```python
from build123d import *

# Parameters (mm, degrees)
SKETCH_W              = 115
SKETCH_H              = 25
PAD_DEPTH             = 3
PAD001_DEPTH          = 3
SKETCH002_W           = 115
SKETCH002_H           = 25
SKETCH002_W_2         = 96
SKETCH002_H_2         = 3
PAD002_DEPTH          = 3
SKETCH003_R           = 1.55
POCKET_DEPTH          = 245.060315
POLARPATTERN_COUNT    = 2
POLARPATTERN001_COUNT = 2
POLARPATTERN002_COUNT = 2
FILLET_R              = 2
SKETCH004_R           = 12.75
POCKET001_DEPTH       = 3
POCKET002_DEPTH       = 3
FILLET001_R           = 0.4
FILLET002_R           = 2


with BuildPart() as part:
    # Sketch → Pad (new body)
    with BuildSketch(Plane.XY):
        Rectangle(SKETCH_W, SKETCH_H)
    extrude(amount=PAD_DEPTH)

    # Sketch001 (on Face6 of Pad) → Pad001 (join)
    with BuildSketch(Plane.XY.offset(3)):
        Polygon((-57.5, 12.5), (57.5, 12.5), (57.5, 4), (50, 4), (50, 5), (-50, 5), (-50, 4), (-57.5, 4), align=None)
        Polygon((-57.5, -12.5), (57.5, -12.5), (57.5, -4), (50, -4), (50, -5), (-50, -5), (-50, -4), (-57.5, -4), align=None)
    extrude(amount=PAD001_DEPTH)

    # Sketch002 (on Face12 of Pad001) → Pad002 (join)
    with BuildSketch(Plane.XY.offset(6)):
        Rectangle(SKETCH002_W, SKETCH002_H)
        Rectangle(SKETCH002_W_2, SKETCH002_H_2, mode=Mode.SUBTRACT)
    extrude(amount=PAD002_DEPTH)

    # Sketch003 (on Face26 of Pad002) → Pocket (cut, through all)
    with BuildSketch(Plane.XY.offset(9)):
        with Locations((-52.5, 7.5)):
            Circle(SKETCH003_R)
    pocket = extrude(amount=-POCKET_DEPTH, mode=Mode.SUBTRACT)

    # PolarPattern: Pocket ×2 about axis
    polarpattern_axis = Axis((0, 0, 0), (0, 1, 0))
    for i in range(1, POLARPATTERN_COUNT):
        add(pocket.rotate(polarpattern_axis, i * 360 / POLARPATTERN_COUNT), mode=Mode.SUBTRACT)

    # PolarPattern001: Pocket ×2 about axis
    polarpattern001_axis = Axis((0, 0, 0), (1, 0, 0))
    for i in range(1, POLARPATTERN001_COUNT):
        add(pocket.rotate(polarpattern001_axis, i * 360 / POLARPATTERN001_COUNT), mode=Mode.SUBTRACT)

    # PolarPattern002: Pocket ×2 about axis
    polarpattern002_axis = Axis((0, 0, 9), (0, 0, 1))
    for i in range(1, POLARPATTERN002_COUNT):
        add(pocket.rotate(polarpattern002_axis, i * 360 / POLARPATTERN002_COUNT), mode=Mode.SUBTRACT)

    # Fillet
    fillet_edges = [part.edges().sort_by_distance(p)[0] for p in [
        (57.5, 12.5, 7.5),
        (57.5, 12.5, 4.5),
        (57.5, 12.5, 1.5),
        (57.5, -12.5, 7.5),
        (-57.5, 12.5, 7.5),
        (-57.5, -12.5, 7.5),
    ]]
    fillet(fillet_edges, radius=FILLET_R)

    # Sketch004 (on Face2 of Fillet) → Pocket001 (cut)
    with BuildSketch(Plane(origin=(0, 0, 0), x_dir=(1, 0, 0), z_dir=(0, 0, -1))):
        with Locations((0, -4.31247)):
            Circle(SKETCH004_R)
    extrude(amount=-POCKET001_DEPTH, mode=Mode.SUBTRACT)

    # Sketch005 (on Face2 of Pocket001) → Pocket002 (cut)
    with BuildSketch(Plane(origin=(0, 0, 0), x_dir=(1, 0, 0), z_dir=(0, 0, -1))):
        Polygon((0.086598, 10.584693), (-50.025204, 10.584693), (-50.025204, 6.371434), (-55.624748, 3.161258), (-55.624748, -3.408425), (-50.493088, -3.376352), (-45.134857, 4.115264), (-43.691578, 5.783052), (0.086598, 5.783052), align=None)
    extrude(amount=-POCKET002_DEPTH, mode=Mode.SUBTRACT)

    # Fillet001
    fillet001_edges = [part.edges().sort_by_distance(p)[0] for p in [
        (-7.787357, -5.783052, 1.5),
    ]]
    fillet(fillet001_edges, radius=FILLET001_R)

    # Fillet002
    fillet002_edges = [part.edges().sort_by_distance(p)[0] for p in [
        (0.086598, -8.437236, 1.5),
    ]]
    fillet(fillet002_edges, radius=FILLET002_R)


solid = part.part
```
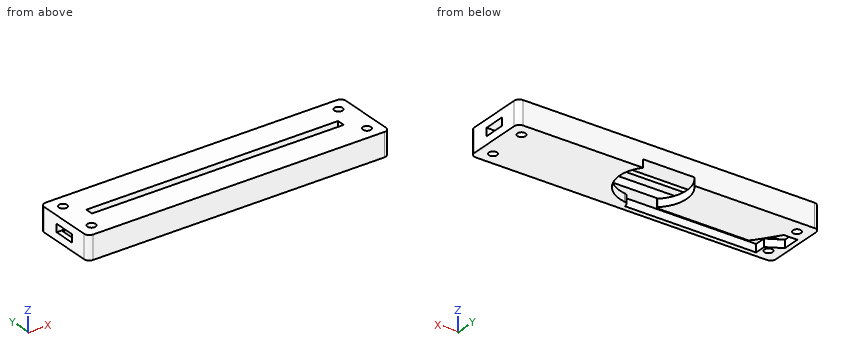
The model under review builds one solid part; all positions refer to its coordinate system, in mm. Give positions to 0.01 mm unless a question says otherwise; leave off trailing zeros. Write each loop counter-clockwise with the first axis right and the second up, starting at its lowest first coordinate (ties: lowest second). Pieces come first, ordered by that corner, then holes. Notation, with made-up numbers: M 19.5,6.25 L 44.5,6.25 A32 ccw 44.5,36.25 Z; hole C 55,24 d7. An arc over 180 degrees is marked long. Write item = value, one per line. Start each with the question number.
Q1. For line 1 (Y direction, x = 52.5, z = 7.25); line 2 (Y direction, x = 52.5, z = 5.25); line 3 (X direction, y = -7.5, z = 5.25), list the stretches that pass through material, from the lowest coordinate up.
Q2. We need section B-B (z = 7.25). State the section outline as (x, y) points, plus the area to 3 significant figures.
Q3. We need section C-C (x = -52.5). State the section outline as (y, z) points, plus the area to 3 significant figures.
Q4. We need section D-D (y = 7.5). State the section outline as (x, z) points.
Q5. We need section A-A (x = 52.5). State the section outline as (y, z) points, plus the area to 3 significant figures.
Q6. Clearance check with a flat-ended pin moving along its axis: pin 1 (8.5 mm diameter, centred on x = 0, y = 9, fed in from -Z). State where the tip first meets the part, or that it passes through.
Result set:
q1.line_1 = -12.5 to -9.05, -5.95 to 5.95, 9.05 to 12.5
q1.line_2 = -12.5 to -9.05, -5.95 to -4, 4 to 5.95, 9.05 to 12.5
q1.line_3 = -57.5 to -54.05, -50.95 to 50.95, 54.05 to 57.5
q2.outline = M -57.5,-10.5 A2 ccw -55.5,-12.5 L 55.5,-12.5 A2 ccw 57.5,-10.5 L 57.5,10.5 A2 ccw 55.5,12.5 L -55.5,12.5 A2 ccw -57.5,10.5 Z; hole C -52.5,-7.5 d3.1; hole C -52.5,7.5 d3.1; hole M -48,-1.5 L 48,-1.5 L 48,1.5 L -48,1.5 Z; hole C 52.5,-7.5 d3.1; hole C 52.5,7.5 d3.1
q2.area = 2,550 mm2
q3.outline = M -12.5,0 L -9.05,0 L -9.05,9 L -12.5,9 Z; M -5.95,0 L -4.95,0 L -4.95,3 L -4,3 L -4,6 L 4,6 L 4,3 L 3.39,3 L 3.39,0 L 5.95,0 L 5.95,9 L -5.95,9 Z; M 9.05,0 L 12.5,0 L 12.5,9 L 9.05,9 Z
q3.area = 120 mm2
q4.outline = M -57.5,0 L -54.05,0 L -54.05,9 L -57.5,9 Z; M -50.95,0 L -12.35,0 L -12.35,3 L 12.35,3 L 12.35,0 L 50.95,0 L 50.95,9 L -50.95,9 Z; M 54.05,0 L 57.5,0 L 57.5,9 L 54.05,9 Z
q5.outline = M -12.5,0 L -9.05,0 L -9.05,9 L -12.5,9 Z; M -5.95,0 L 5.95,0 L 5.95,9 L -5.95,9 Z; M 9.05,0 L 12.5,0 L 12.5,9 L 9.05,9 Z; hole M -4,3 L 4,3 L 4,6 L -4,6 Z
q5.area = 145 mm2
q6.pin_1 = 3
